Autodesk Inventor part; units mm, degrees
ref_plane "YZ Plane" through (0, 0, 0) normal (1, 0, 0) x (0, 1, 0)
ref_plane "XZ Plane" through (0, 0, 0) normal (0, 1, 0) x (-1, 0, 0)
ref_plane "XY Plane" through (0, 0, 0) normal (0, 0, 1) x (1, 0, 0)
sketch "Sketch1" plane through (0, 0, 0) normal (0, 1, 0) x (-1, 0, 0)
  line L0 (39.5135, 44.2255) -> (0.0135, 44.2255)
  line L1 (0.0135, 44.2255) -> (0.0135, -52.7745)
  line L2 (0.0135, -52.7745) -> (39.5135, -52.7745)
  line L3 (39.5135, -52.7745) -> (39.5135, 44.2255)
  point P0 (0, 0)
  dimension "LCD_Screen_Width" = 97
  dimension "LCD_Screen_Height" = 39.5
extrude "Extrusion1" add sketch "Sketch1" along normal blind 9.9
sketch "Sketch2" plane through (0, 9.9, 0) normal (0, 1, 0) x (1, 0, 0)
  line L0 (-32.7635, -33.7255) -> (-6.7635, -33.7255)
  line L1 (-6.7635, -33.7255) -> (-6.7635, 42.2745)
  line L2 (-6.7635, 42.2745) -> (-32.7635, 42.2745)
  line L3 (-32.7635, 42.2745) -> (-32.7635, -33.7255)
  line L4 (-39.5135, 52.7745) -> (-39.5135, -44.2255) construction
  line L5 (-39.5135, 4.2745) -> (-32.7635, 4.2745) construction
  line L6 (-6.7635, 4.2745) -> (-0.0135, 4.2745) construction
  line L7 (-0.0135, -44.2255) -> (-0.0135, 52.7745) construction
  point P0 (0, 0)
  dimension "LCD_Viewable_Height" = 26
  dimension "LCD_Viewable_Width" = 76
extrude "Extrusion2" cut sketch "Sketch2" against normal blind 1
sketch "Sketch3" plane through (0, 0, 0) normal (0, -1, 0) x (1, 0, 0)
  line L0 (-0.0135, 44.2255) -> (-0.2635, 44.2255)
  line L1 (-0.2635, 44.2255) -> (-0.2635, 40.2255)
  line L2 (-0.2635, 40.2255) -> (-0.0135, 40.2255)
  line L3 (-0.0135, 40.2255) -> (-0.0135, 44.2255)
  line L4 (-0.0135, -2.2745) -> (-0.2635, -2.2745)
  line L5 (-0.2635, -2.2745) -> (-0.2635, -6.2745)
  line L6 (-0.2635, -6.2745) -> (-0.0135, -6.2745)
  line L7 (-0.0135, -6.2745) -> (-0.0135, -2.2745)
  line L8 (-0.0135, -48.7745) -> (-0.2635, -48.7745)
  line L9 (-0.2635, -48.7745) -> (-0.2635, -52.7745)
  line L10 (-0.2635, -52.7745) -> (-0.0135, -52.7745)
  line L11 (-0.0135, -52.7745) -> (-0.0135, -48.7745)
  line L12 (-39.2635, -48.7745) -> (-39.5135, -48.7745)
  line L13 (-39.5135, -48.7745) -> (-39.5135, -52.7745)
  line L14 (-39.5135, -52.7745) -> (-39.2635, -52.7745)
  line L15 (-39.2635, -52.7745) -> (-39.2635, -48.7745)
  line L16 (-39.2635, -2.2745) -> (-39.5135, -2.2745)
  line L17 (-39.5135, -2.2745) -> (-39.5135, -6.2745)
  line L18 (-39.5135, -6.2745) -> (-39.2635, -6.2745)
  line L19 (-39.2635, -6.2745) -> (-39.2635, -2.2745)
  line L20 (-39.2635, 44.2255) -> (-39.5135, 44.2255)
  line L21 (-39.5135, 44.2255) -> (-39.5135, 40.2255)
  line L22 (-39.5135, 40.2255) -> (-39.2635, 40.2255)
  line L23 (-39.2635, 40.2255) -> (-39.2635, 44.2255)
  line L24 (-0.0135, 44.2255) -> (-0.0135, -52.7745)
  line L25 (-39.5135, -52.7745) -> (-39.5135, 44.2255)
  line L26 (-39.5135, 44.2255) -> (-0.0135, 44.2255)
  line L27 (-0.0135, -52.7745) -> (-39.5135, -52.7745)
  line L28 (-0.2635, 40.2255) -> (-0.2635, -2.2745) construction
  line L29 (-0.2635, -6.2745) -> (-0.2635, -48.7745) construction
  point P0 (0, 0)
  dimension "LCD_Screen_Tab_Width" = 0.25
  dimension "LCD_Screen_Tab_Length" = 4
extrude "Extrusion3" add sketch "Sketch3" along normal blind 4.1 contours L3 L2 L1 L0 | L23 L22 L21 L20 | L7 L6 L5 L4 | L11 L10 L9 L8 | L16 L19 L18 L17 | L12 L15 L14 L13
properties part number "LCD_Screen" material "Steel, Mild"
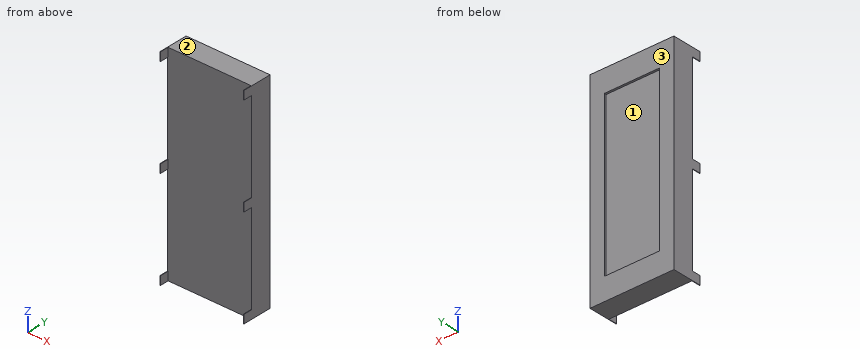
Part model, mm, in its own coordinate system. Face numbers are marked on the shaded views. Give positions to 0.01 mm unless a question says otherwise; leave off trailing zeros. Order: outer loops, then holes, each group sorted by start corner. A loop starts at its lowest first (then second) coordinate and runs counter-clockwise, first axis right, second up. Notation, with made-up numbers: (-12, 40) - (-5, 40) arc R9 ccw to (-5, 50) - close; hole circle Ø7 at (-14.5, 84.5). An arc over 180 degrees is marked (long way). One line per question, with ' | ' between items.
1. Drop flat-ended pins along their axis: P1, Ø5, axis at x = -26, z = -27, coming from the +Y side; P2, Ø12, axis at x = -15, z = 6, coming from the -Y side; P3, Ø5, axis at x = -4.5, y = -0.5, coming from the -Z side. Give the stop position or say it passes through.
Filled in:
P1: y = 8.9 | P2: y = 0 | P3: z = -52.77
2. Band-saw the part on D-D on z = 37.5. List the corners of the cut face in (x, y), then the cut area to 3 significant figures.
Filled in:
outline: (-39.51, 0) - (-0.01, 0) - (-0.01, 9.9) - (-39.51, 9.9) - close | area: 391 mm²
3. Band-saw the part on C-C on z = -30.5. List the corners of the cut face in (x, y).
Filled in:
outline: (-39.51, 0) - (-0.01, 0) - (-0.01, 9.9) - (-6.76, 9.9) - (-6.76, 8.9) - (-32.76, 8.9) - (-32.76, 9.9) - (-39.51, 9.9) - close
4. Pull direction Z, two halves, no side cores. Call the marked faces 1, 2 and 3: +Z half, -Z half, draft (parallel to the pull), parting line (faces both ways), or undercut.
Filled in:
face 1: undercut | face 2: +Z half | face 3: draft
5. Drill centre lines: probe 1 along Y at (x, z) = (-38, -1); probe 2 along X at (y, z) = (-1.5, -4); probe 3 along Y at (x, z) = (-12, -18). Where is each one in solid material? Low to high.
Filled in:
probe 1: 0 to 9.9 | probe 2: -39.51 to -39.26, -0.26 to -0.01 | probe 3: 0 to 8.9
6. Band-saw the part on B-B on x = -30. List the corners of the cut face in (y, z).
Filled in:
outline: (0, -52.77) - (9.9, -52.77) - (9.9, -42.27) - (8.9, -42.27) - (8.9, 33.73) - (9.9, 33.73) - (9.9, 44.23) - (0, 44.23) - close
7. Band-saw the part on A-A on y = -2.25. List the corners of the cut face in (x, z), then the cut area to 3 significant figures.
Filled in:
outline: (-39.51, -52.77) - (-39.26, -52.77) - (-39.26, -48.77) - (-39.51, -48.77) - close; (-39.51, -6.27) - (-39.26, -6.27) - (-39.26, -2.27) - (-39.51, -2.27) - close; (-39.51, 40.23) - (-39.26, 40.23) - (-39.26, 44.23) - (-39.51, 44.23) - close; (-0.26, -52.77) - (-0.01, -52.77) - (-0.01, -48.77) - (-0.26, -48.77) - close; (-0.26, -6.27) - (-0.01, -6.27) - (-0.01, -2.27) - (-0.26, -2.27) - close; (-0.26, 40.23) - (-0.01, 40.23) - (-0.01, 44.23) - (-0.26, 44.23) - close | area: 6.00 mm²
